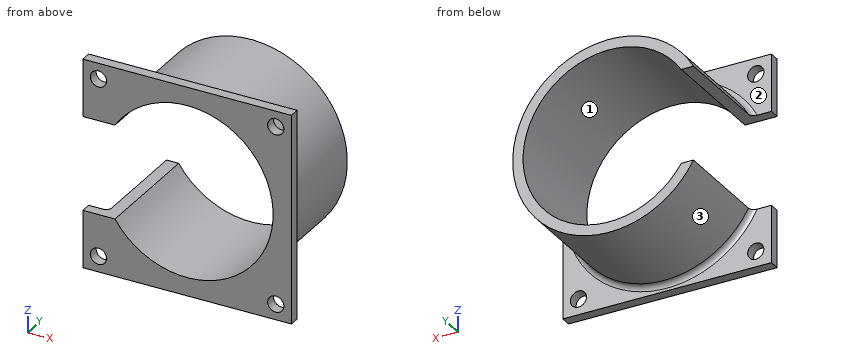
```python
from build123d import *

# Parameters (mm, degrees)
SKETCH_1_W          = 40
SKETCH_1_H          = 40
SKETCH_1_R          = 1.55
SKETCH_1_R_2        = 16.5
EXTRUDE_1_DEPTH     = 2
SKETCH_2_R          = 18.5
SKETCH_2_R_2        = 16.5
EXTRUDE_2_DEPTH     = 20
FILLET_1_R          = 1
CUT_EXTRUDE_1_DEPTH = 36.832945734


with BuildPart() as part:
    # 草图1 → 凸台-拉伸1 (new body)
    with BuildSketch(Plane(origin=(0, 0, 0), x_dir=(1, 0, 0), z_dir=(0, 1, 0))):
        Rectangle(SKETCH_1_W, SKETCH_1_H)
        with Locations(Location((-17, 17, 0), (0, 0, 270))):
            Circle(SKETCH_1_R, mode=Mode.SUBTRACT)
        with Locations(Location((17, 17, 0), (0, 0, 270))):
            Circle(SKETCH_1_R, mode=Mode.SUBTRACT)
        with Locations(Location((17, -17, 0), (0, 0, 270))):
            Circle(SKETCH_1_R, mode=Mode.SUBTRACT)
        with Locations(Location((-17, -17, 0), (0, 0, 270))):
            Circle(SKETCH_1_R, mode=Mode.SUBTRACT)
        with Locations(Location((0, 0, 0), (0, 0, 270))):
            Circle(SKETCH_1_R_2, mode=Mode.SUBTRACT)
    extrude(amount=EXTRUDE_1_DEPTH)

    # 草图2 → 凸台-拉伸2 (add)
    with BuildSketch(Plane(origin=(0, 2, 0), x_dir=(1, 0, 0), z_dir=(0, 1, 0))):
        with Locations(Location((0, 0, 0), (0, 0, 270))):
            Circle(SKETCH_2_R)
        with Locations(Location((0, 0, 0), (0, 0, 270))):
            Circle(SKETCH_2_R_2, mode=Mode.SUBTRACT)
    extrude(amount=EXTRUDE_2_DEPTH)

    # 圆角1
    fillet_1_edges = [part.edges().sort_by_distance(p)[0] for p in [
        (0, 2, -18.5),
    ]]
    fillet(fillet_1_edges, radius=FILLET_1_R)

    # 草图3 → 切除-拉伸1 (cut, through all)
    with BuildSketch(Plane.XZ):
        with BuildLine():
            ThreePointArc((-13.829316686, -9), (-15.818244614, -4.693946883), (-16.5, 0))
            ThreePointArc((-16.5, 0), (-15.818244614, 4.693946883), (-13.829316686, 9))
            Line((-13.829316686, 9), (-20, 9))
            Line((-20, 9), (-20, -9))
            Line((-20, -9), (-13.829316686, -9))
        make_face()
    extrude(amount=-CUT_EXTRUDE_1_DEPTH, mode=Mode.SUBTRACT)


solid = part.part
```
Here's how the part is built. I have some questions about the finished solid (model axes, mm). Face numbers are marked on the shaded views. Coordinates: 2 decimals unless noted, no trailing zeros. Order: outer loops, then holes, each group sorted by start corner. A loop starts at its lowest first (then second) coordinate and runs counter-clockwise, first axis right, second up.
1) Imagine slicing it at B-B on z = 0. List the corners of the cut face in (x, y) for me.
2) Will these pins go through, and if not, where does the flat tip stop? pin 1 (2 mm diameter, centred on y = 12, z = 15.5, fed in from -X); pin 2 (2 mm diameter, centred on x = -0.5, y = 8.5, fed in from +Z); pin 3 (1 mm diameter, centred on x = -7.5, y = 13.5, fed in from +Z).
3) Imagine slicing it at C-C on z = 17. State how many separate pieces and enclosed holes the cut face has, and give its area (3 significant figures).
4) I need wall thicknesses on line 1 (X direction, y = 0.8, z = -17); line 2 (X direction, y = 13, z = 0); line 3 (Z direction, x = 15, y = 16). Which ranges of each line are inside material? Lowest first, please.
5) Imagine slicing it at A-A on x = 0. List the corners of the cut face in (y, z) for me, and give its area (3 significant figures).
6) We'd pull the mould along Z, two halves only. Please class the marked faces 1, 2 and 3: +Z half, -Z half, draft (parallel to the pull), parting line (faces both ways), or undercut.
Response values:
1. outline: (16.5, 0) - (20, 0) - (20, 2) - (19.5, 2) arc R1 cw to (18.5, 3) - (18.5, 22) - (16.5, 22) - close
2. pin 1: stops at x = -11.49
2. pin 2: stops at z = 18.5
2. pin 3: stops at z = 17.12
3. separate pieces: 3
3. enclosed holes: 0
3. area: 361 mm2
4. line 1: x = -20 to -18.55, -15.45 to 15.45, 18.55 to 20
4. line 2: x = 16.5 to 18.5
4. line 3: z = -10.83 to -6.87, 6.87 to 10.83
5. outline: (0, -20) - (2, -20) - (2, -19.5) arc R1 cw to (3, -18.5) - (22, -18.5) - (22, -16.5) - (0, -16.5) - close; (0, 16.5) - (22, 16.5) - (22, 18.5) - (3, 18.5) arc R1 cw to (2, 19.5) - (2, 20) - (0, 20) - close
5. area: 94.4 mm2
6. face 1: undercut
6. face 2: draft
6. face 3: parting line
